```python
from build123d import *

# Parameters (mm, degrees)
SKETCH1_W               = 70
SKETCH1_H               = 41
SKETCH1_R               = 4.5
BOSS_EXTRUDE1_DEPTH     = 5
SKETCH2_W               = 5
SKETCH2_H               = 41
BOSS_EXTRUDE2_DEPTH     = 25
BOSS_EXTRUDE3_DEPTH     = 5
CUT_EXTRUDE2_DEPTH      = 61.582588258
CUT_EXTRUDE2_DEPTH_BACK = 61.582588258
SKETCH6_R               = 20
BOSS_EXTRUDE4_DEPTH     = 5
SKETCH7_R               = 4
CUT_EXTRUDE3_DEPTH      = 71.859014952
FILLET1_R               = 2.5


with BuildPart() as part:
    # Sketch1 → Boss-Extrude1 (new body)
    with BuildSketch(Plane.XY):
        Rectangle(SKETCH1_W, SKETCH1_H)
        with Locations((-27, 12.5)):
            Circle(SKETCH1_R, mode=Mode.SUBTRACT)
        with Locations((-27, -12.5)):
            Circle(SKETCH1_R, mode=Mode.SUBTRACT)
        with Locations((27, 12.5)):
            Circle(SKETCH1_R, mode=Mode.SUBTRACT)
        with Locations((27, -12.5)):
            Circle(SKETCH1_R, mode=Mode.SUBTRACT)
    extrude(amount=BOSS_EXTRUDE1_DEPTH)

    # Sketch2 → Boss-Extrude2 (add)
    with BuildSketch(Plane.XY.offset(5)):
        with Locations((-12.5, 0)):
            Rectangle(SKETCH2_W, SKETCH2_H)
        with Locations((12.5, 0)):
            Rectangle(SKETCH2_W, SKETCH2_H)
    extrude(amount=BOSS_EXTRUDE2_DEPTH)

    # Sketch5 → Boss-Extrude3 (add)
    with BuildSketch(Plane.XZ.offset(20.5)):
        with BuildLine():
            Line((-15, 30), (-15, 5))
            Line((-15, 5), (15, 5))
            Line((15, 5), (15, 30))
            ThreePointArc((15, 30), (0, 45), (-15, 30))
        make_face()
    extrude(amount=-BOSS_EXTRUDE3_DEPTH)

    # Sketch3 → Cut-Extrude2 (cut, two sides: drawn at the far end of the back side and taken through both)
    with BuildSketch(Plane(origin=(0, 0, 0), x_dir=(0, 0, -1), z_dir=(1, 0, 0)).offset(-CUT_EXTRUDE2_DEPTH_BACK)):
        Polygon((-5, 20.5), (-30, -15.5), (-49.542972481, -15.5), (-49.542972481, 23.944363396), (-5, 23.944363396), align=None)
    extrude(amount=CUT_EXTRUDE2_DEPTH + CUT_EXTRUDE2_DEPTH_BACK, mode=Mode.SUBTRACT)

    # Sketch6 → Boss-Extrude4 (add)
    with BuildSketch(Plane.XZ.offset(20.5)):
        with Locations(Location((0, 30, 0), (0, 0, 221.409622109))):
            Circle(SKETCH6_R)
    extrude(amount=BOSS_EXTRUDE4_DEPTH)

    # Sketch7 → Cut-Extrude3 (cut, through all)
    with BuildSketch(Plane(origin=(0, -15.5, 0), x_dir=(1, 0, 0), z_dir=(0, 1, 0))):
        with Locations(Location((0, -30, 0), (0, 0, 180))):
            Circle(SKETCH7_R)
    extrude(amount=-CUT_EXTRUDE3_DEPTH, mode=Mode.SUBTRACT)

    # Fillet1
    # the kernel refuses this fillet: 2.5 mm, written as the material it adds along each edge
    with BuildSketch(Plane(origin=(-15, -20.5, 10.521243445), x_dir=(0, 1, 0), z_dir=(0, 0, 1))) as fillet1_piece_1_section:
        with BuildLine():
            CenterArc((FILLET1_R, FILLET1_R), FILLET1_R, 180, 90)
            Line((0, FILLET1_R), (0, 0))
            Line((0, 0), (FILLET1_R, 0))
        make_face()
    fillet1_piece_1 = extrude(amount=19.478756555, mode=Mode.PRIVATE)
    fillet1_piece_1 = fillet1_piece_1 & Plane(origin=(0, -19.928453247, 30), x_dir=(-0.7500000000031269, 0, -0.6614378277626021), z_dir=(0, 1, 0)) * Cylinder(20, 49, mode=Mode.PRIVATE)
    add(fillet1_piece_1)
    with BuildSketch(Plane(origin=(15, -20.5, 10.521243445), x_dir=(0, 1, 0), z_dir=(0, 0, 1))) as fillet1_piece_2_section:
        with BuildLine():
            CenterArc((FILLET1_R, -FILLET1_R), FILLET1_R, 90, 90)
            Line((0, -FILLET1_R), (0, 0))
            Line((0, 0), (FILLET1_R, 0))
        make_face()
    fillet1_piece_2 = extrude(amount=19.478756555, mode=Mode.PRIVATE)
    fillet1_piece_2 = fillet1_piece_2 & Plane(origin=(0, -19.928453234, 30), x_dir=(-0.7500000000031269, 0, -0.6614378277626021), z_dir=(0, 1, 0)) * Cylinder(20, 49, mode=Mode.PRIVATE)
    add(fillet1_piece_2)
    with BuildSketch(Plane(origin=(0, -20.5, 30), x_dir=(1, 0, 0), z_dir=(0, 0, -1))) as fillet1_piece_3:
        with BuildLine():
            CenterArc((15 + FILLET1_R, -FILLET1_R), FILLET1_R, 90, 90)
            Line((15, -FILLET1_R), (15, 0))
            Line((15, 0), (15 + FILLET1_R, 0))
        make_face()
    revolve(axis=Axis((0, -20.5, 30), (0, -1, 0)), revolution_arc=180)


solid = part.part
```
Input: part model. Units: mm. Frame: model coordinates. A direction names the side the tool comes from. Coordinates: 2 decimals unless noted, no trailing zeros. Loops run counter-clockwise (first coordinate to the right, second up) from the corner with the lowest first, then second, coordinate; pieces in that order, holes last. Notation, with made-up numbers: (-26.75, -22) -> (-13.75, -22) arc R10 ccw to (-13.75, -5) -> close; hole circle Ø11 at (-34, -8). An arc over 180 degrees is marked (long way). Use a Markdown table: item, result.
1) Access query for faces 1 (the flat face through (0, 20.5, 2)), 2 (the flat face through (-10, -2, 15)), 3 (the cylindrical face through (-16, -20, 23)). Directions: +Z, -Z, +X, -X, +Y, -Y. A direction counts if a zero-diameter tool reaches every point of the face in a straight line with its end or side. Return the directions, or none.
Results found:
| item | result |
|---|---|
| face 1 | +Z, -Z, +X, -X, +Y |
| face 2 | +Z, +Y |
| face 3 | +Z, -X, +Y |
2) Cut plane B-B (y = 9.5). Return the cut outline in (x, z), then the cut area to 3 significant figures.
Results found:
| item | result |
|---|---|
| outline | (-35, 0) -> (-30.35, 0) -> (-30.35, 5) -> (-35, 5) -> close; (-23.65, 0) -> (23.65, 0) -> (23.65, 5) -> (15, 5) -> (15, 12.64) -> (10, 12.64) -> (10, 5) -> (-10, 5) -> (-10, 12.64) -> (-15, 12.64) -> (-15, 5) -> (-23.65, 5) -> close; (30.35, 0) -> (35, 0) -> (35, 5) -> (30.35, 5) -> close |
| area | 359 mm2 |
3) Pull-direction query (Y, two-part tool) for faces 4 (the flat face through (0, 0, 0)), 5 (the cylindrical face through (26.41, -8.04, 2.46)), 6 (the flat face through (-12.535, 2.752, 17.325)); classes: released by +Y, released by -Y, zero draft, split by the parting line, or undercut.
Results found:
| item | result |
|---|---|
| face 4 | zero draft |
| face 5 | undercut |
| face 6 | released by +Y |
4) Cut plane A-A (x = 0). Return the cut outline in (y, z).
Results found:
| item | result |
|---|---|
| outline | (-25.5, 10) -> (-20.5, 10) -> (-20.5, 0) -> (20.5, 0) -> (20.5, 5) -> (-15.5, 5) -> (-15.5, 26) -> (-25.5, 26) -> close; (-25.5, 34) -> (-15.5, 34) -> (-15.5, 45) -> (-18, 45) arc R2.5 cw to (-20.5, 47.5) -> (-20.5, 50) -> (-25.5, 50) -> close |
5) Cut plane D-D (x = 26). Return the cut outline in (y, z), then the cut area to 3 significant figures.
Results found:
| item | result |
|---|---|
| outline | (-20.5, 0) -> (-16.89, 0) -> (-16.89, 5) -> (-20.5, 5) -> close; (-8.11, 0) -> (8.11, 0) -> (8.11, 5) -> (-8.11, 5) -> close; (16.89, 0) -> (20.5, 0) -> (20.5, 5) -> (16.89, 5) -> close |
| area | 117 mm2 |
6) Material intervals for line 1 along Y through (x, z) = (-27, 2); line 2 along X through (y, z) = (2.5, 15.5); line 3 along X through (y, z) = (-12, 1), sorted ascending. Write a range as from..to.
Results found:
| item | result |
|---|---|
| line 1 | y = -20.5..-17, -8..8, 17..20.5 |
| line 2 | x = -15..-10, 10..15 |
| line 3 | x = -35..-31.47, -22.53..22.53, 31.47..35 |
7) Contact query for flat-ended pins moving along their axis: pin 1 (10 mm diameter, centred on x = -27.5, y = -16, fed in from +Z); pin 2 (22 mm diameter, centred on x = -2.5, y = -5, fed in from +Z); pin 3 (8 mm diameter, centred on y = -1, z = 10, fed in from +X); pin 4 (11.5 mm diameter, centred on x = 27, y = -12.5, fed in from -Z). Output: stop coordinate, or through.
Results found:
| item | result |
|---|---|
| pin 1 | stops at z = 5 |
| pin 2 | stops at z = 45 |
| pin 3 | stops at x = 15 |
| pin 4 | stops at z = 0 |
8) Cut plane C-C (z = 27.5). Return the cut outline in (x, y).
Results found:
| item | result |
|---|---|
| outline | (-19.84, -25.5) -> (-3.12, -25.5) -> (-3.12, -15.5) -> (-10, -15.5) -> (-10, -11.9) -> (-15, -11.9) -> (-15, -18) arc R2.5 cw to (-17.5, -20.5) -> (-19.84, -20.5) -> close; (3.12, -25.5) -> (19.84, -25.5) -> (19.84, -20.5) -> (17.5, -20.5) arc R2.5 cw to (15, -18) -> (15, -11.9) -> (10, -11.9) -> (10, -15.5) -> (3.12, -15.5) -> close |
